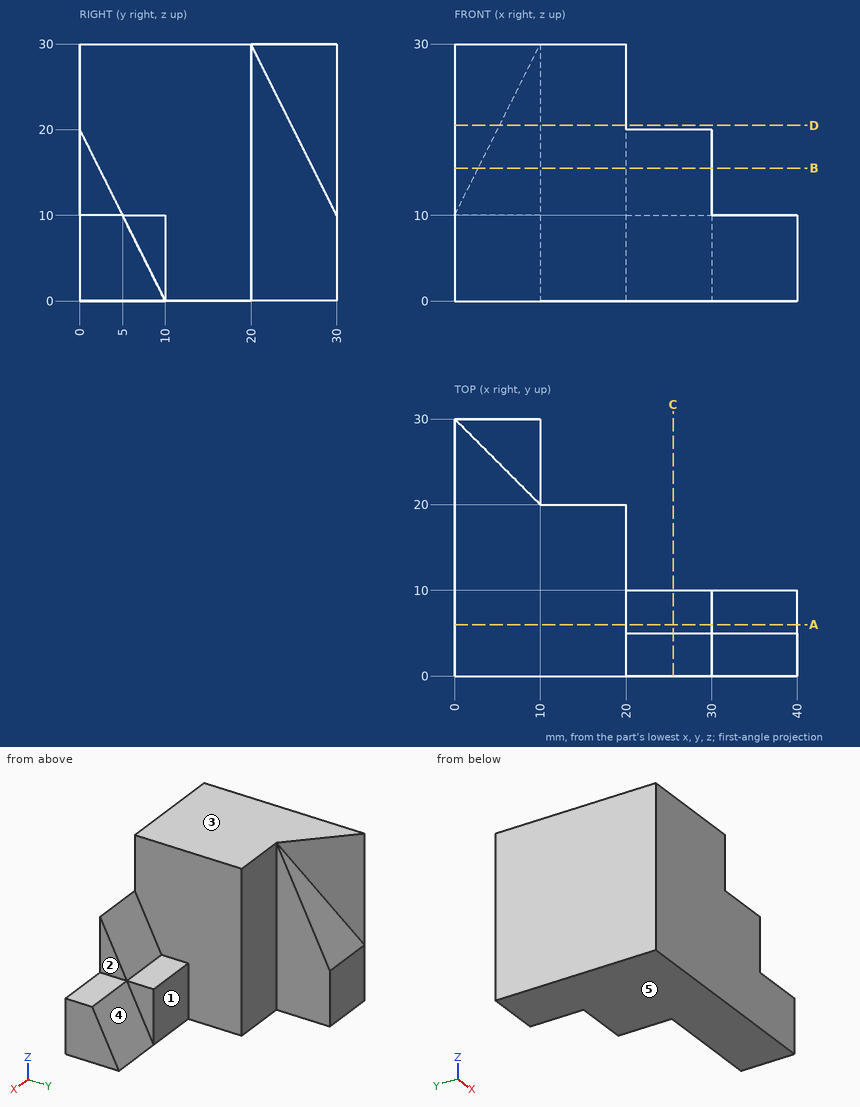
Source: three-view drawing plus pictorial views. Frame: mm from the lowest corner of the part. A direction names the side the tool comes from. Round coordinates to 2 decimals unless told otherwise and drop trailing zeros. Loops run counter-clockwise (first coordinate to the right, second up) from the corner with the lowest first, then second, coordinate; pieces in that order, holes last. Notation, with made-up numbers: M 36,-19 L 65,-19 A24 ccw 65,-6 Z; hole C 25,47.25 d5. An arc over 180 degrees is marked long. Put each result on its own line as item: value. Start each with the question number.
(1) Section query A-A (y = 6). Return loops of the section in (x, z).
(2) Section query C-C (x = 25.5). Return loops of the section in (y, z), then the cut area to 3 significant figures.
(3) Contact query for flat-ended pins moving along their axis: pin 1 Ø1.5 at (x, y) = (33, 3) entering from +Z; pin 2 Ø12 at (x, z) = (23, 8.5) entering from +Y; pin 3 Ø3 at (y, z) = (25.5, 16) entering from +X. Output: stop coordinate, or through.
(4) Set-up query: the marked faces 1, 2, 3, 4 and 5. Return all of +Z, -Z, +X, -X, +Y, -Y with unobstructed straight access to the full face (end or side cutting, diameter ignored); none if empty.
(5) Section query B-B (z = 15.5). Return loops of the section in (x, y), then the cut area to 3 significant figures.
(6) Section query D-D (z = 20.5). Return loops of the section in (x, y).
(7) Material intervals for line 1 along X through (y, z) = (17, 5); line 2 along X through (y, z) = (26.5, 10.5), sorted ascending. Write a range as [from, to].
Findings below:
1. outline: M 0,0 L 40,0 L 40,8 L 30,8 L 30,10 L 20,10 L 20,30 L 0,30 Z
2. outline: M 0,0 L 10,0 L 10,10 L 5,10 L 0,20 Z
2. area: 125 mm2
3. pin 1: stops at z = 10
3. pin 2: stops at y = 20
3. pin 3: stops at x = 10
4. face 1: +Z, -Z, +X, +Y
4. face 2: +Z, +X, +Y, -Y
4. face 3: +Z, +X, -X, +Y, -Y
4. face 4: +Z, +X, +Y
4. face 5: -Z, +X, -X, +Y, -Y
5. outline: M 0,0 L 30,0 L 30,2.25 L 20,2.25 L 20,20 L 10,20 L 10,27.25 L 2.75,27.25 L 0,30 Z
5. area: 499 mm2
6. outline: M 0,0 L 20,0 L 20,20 L 10,20 L 10,24.75 L 5.25,24.75 L 0,30 Z
7. line 1: x = [0, 20]
7. line 2: x = [0, 10]
